Part model, mm, in its own coordinate system. Give positions to 0.01 mm unless a question says otherwise; leave off trailing zeros. Write each loop counter-clockwise with the first axis right and the second up, starting at its lowest first coordinate (ties: lowest second). Pieces come first, ordered by that corner, then holes.
```python
from build123d import *

# Parameters (mm, degrees)
F0_W     = 304.8
F0_H     = 177.8
F1_DEPTH = 3.175
F3_D     = 5.1054
F4_D     = 19.05


with BuildPart() as f1:
    # F0 (on Top) → F1 (new body)
    with BuildSketch(Plane.XY):
        with Locations((4.422663, 18.39034)):
            Rectangle(F0_W, F0_H)
    extrude(amount=F1_DEPTH)

    # F3 (through all)
    with Locations(Plane.XY.offset(3.175)):
        with Locations((-33.677337, -32.40966), (-33.677337, 94.59034), (-33.677337, 43.79034), (-8.277337, 43.79034), (-33.677337, -57.80966), (-8.277337, 18.39034), (-8.277337, -7.00966), (-8.277337, -57.80966), (-84.477337, 94.59034), (-8.277337, 94.59034), (-8.277337, -32.40966), (-59.077337, 69.19034), (-33.677337, 18.39034), (-59.077337, 94.59034), (-33.677337, -7.00966), (-8.277337, 69.19034), (-84.477337, 69.19034), (-33.677337, 69.19034), (-135.277337, 43.79034), (-135.277337, 18.39034), (-109.877337, -32.40966), (-109.877337, 43.79034), (-109.877337, -57.80966), (-135.277337, -57.80966), (-109.877337, -7.00966), (-135.277337, -32.40966), (-109.877337, 18.39034), (-135.277337, -7.00966)):
            Hole(F3_D / 2)

    # F4 (through all)
    with Locations(Plane.XY.offset(3.175)):
        with Locations((-122.577337, 81.89034)):
            Hole(F4_D / 2)


solid = f1.part
```
1) Saw through at B-B, the plane y = 77. Write the cut outline in (x, z) (3 decimals).
Answers follow:
outline: (-147.977, 0) - (-130.751, 0) - (-130.751, 3.175) - (-147.977, 3.175) - close; (-114.404, 0) - (156.823, 0) - (156.823, 3.175) - (-114.404, 3.175) - close
2) Saw through at A-A, the plane z = 1.5. Count the separate pieces of the cut face and the enclosed holes in it, then the cut area to 3 significant figures.
Answers follow:
separate pieces: 1
enclosed holes: 29
area: 53,300 mm2
3) Pin check, flat tip, straight feed: pin 1 Ø3 at (x, y) = (-109.88, 43.79) entering from -Z. Stop position of the tip, or through.
Answers follow:
pin 1: passes through
4) Wall check: L1, parallel to X at y = -6.5, z = 0.7; L2, parallel to Y at x = -59, z = 2.1; L3, parallel to Y at x = -118, z = 1.65. Give the ranges that are in metal, low to high.
Answers follow:
L1: x = -147.98 to -137.78, -132.78 to -112.38, -107.38 to -36.18, -31.18 to -10.78, -5.78 to 156.82
L2: y = -70.51 to 66.64, 71.74 to 92.04, 97.14 to 107.29
L3: y = -70.51 to 73.54, 90.24 to 107.29
5) Two-plate mould, pull along X, no slides. Class faces 1 (the face through (-113.06, 82.31, 1.57)), 2 (the face through (2, 20, 3.175)): +X half, -X half, draft (parallel to the pull), parting line (faces both ways), or undercut.
Answers follow:
face 1: undercut
face 2: draft
